Print and shaded views of the part. All mm, measured from the part's lowest x, y and z. Round coordinates to 2 decimals unless told otherwise and drop trailing zeros. Loops run counter-clockwise (first coordinate to the right, second up) from the corner with the lowest first, then second, coordinate; pieces in that order, holes last. Notation, with made-up numbers: (88.25, -28.75) - (106.25, -28.75) arc R32 cw to (106.25, 6.25) - close; hole circle Ø11 at (-35.5, -20). An arc over 180 degrees is marked (long way). Answer as a JSON object with one key per item and string values.
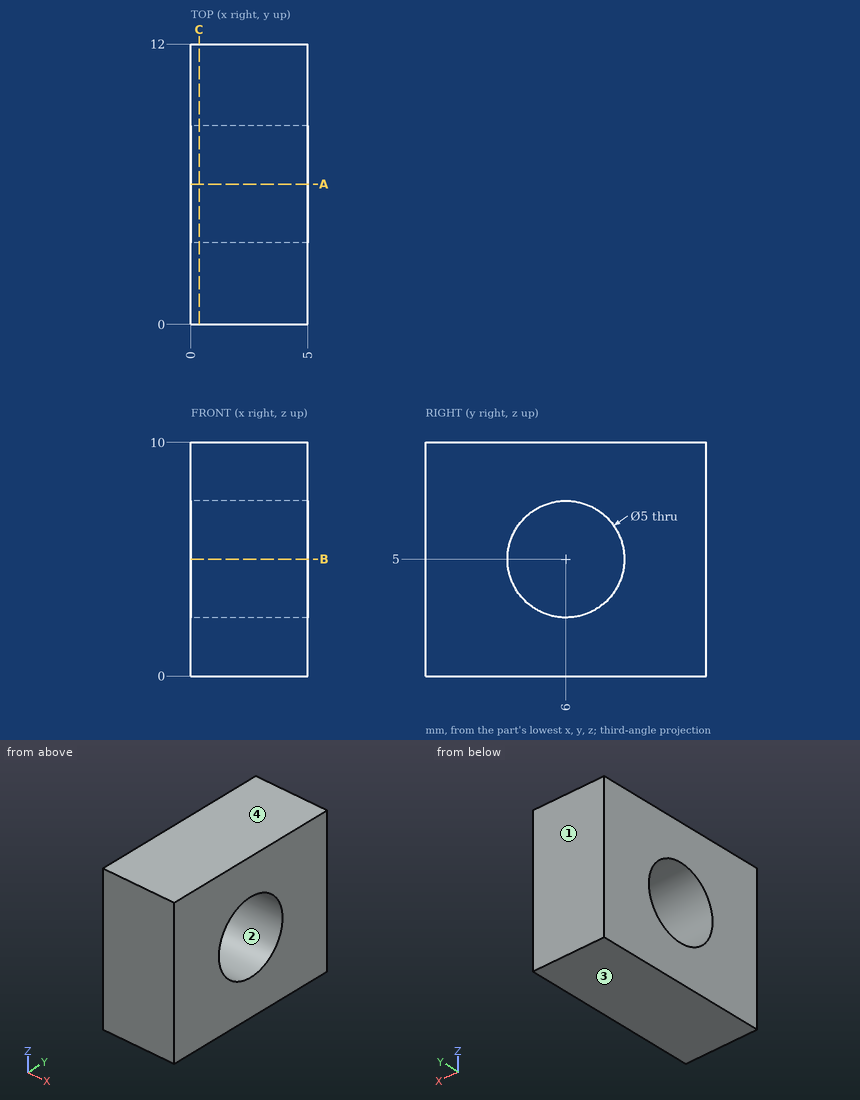
1) Drop a flat-ended pin along its axis: P1, Ø1, axis at y = 2, z = 2.5, coming from the -X side. Give the stop position or say it passes through.
Values follow:
{"P1": "x = 0"}
2) Slice it at B-B on z = 5. List the corners of the cut face in (x, y).
Values follow:
{"outline": "(0, 0) - (5, 0) - (5, 3.5) - (0, 3.5) - close; (0, 8.5) - (5, 8.5) - (5, 12) - (0, 12) - close"}
3) Two-plate mould, pull along Z, no slides. Class the marked faces 1, 2, 3 and 4: pulls with the +Z half, pulls with the -Z half, needs draft (parallel to the pull), parting line crosses it, or undercut.
Values follow:
{"face 1": "needs draft", "face 2": "undercut", "face 3": "pulls with the -Z half", "face 4": "pulls with the +Z half"}
4) Slice it at A-A on y = 6. List the corners of the cut face in (x, z).
Values follow:
{"outline": "(0, 0) - (5, 0) - (5, 2.5) - (0, 2.5) - close; (0, 7.5) - (5, 7.5) - (5, 10) - (0, 10) - close"}
5) Slice it at C-C on x = 0.35. List the corners of the cut face in (y, z), then the cut area to 3 significant figures.
Values follow:
{"outline": "(0, 0) - (12, 0) - (12, 10) - (0, 10) - close; hole circle Ø5 at (6, 5)", "area": "100 mm²"}
6) Probe probe 1 along Z at (x, y) = (3.55, 6); probe 2 along Z at (x, y) = (3.2, 8.25); probe 3 along Y at (x, z) = (3.9, 4). List the from-to ranges inside material, lowest first.
Values follow:
{"probe 1": "0 to 2.5, 7.5 to 10", "probe 2": "0 to 3.91, 6.09 to 10", "probe 3": "0 to 3.71, 8.29 to 12"}
